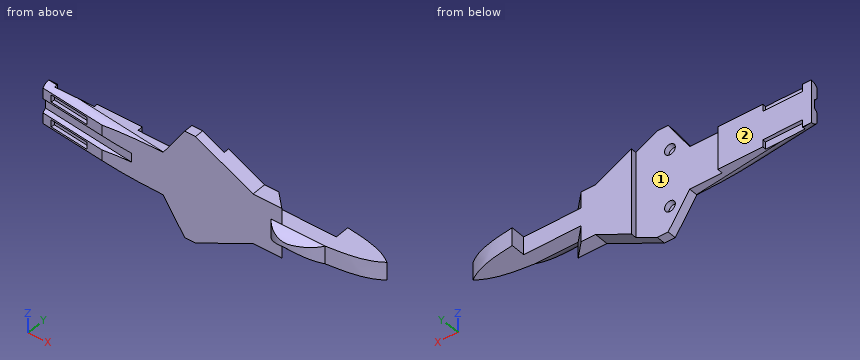
```python
from build123d import *

# Parameters (mm, degrees)
BOSS_EXTRUDE1_DEPTH     = 4
SKETCH2_R               = 1.5
BOSS_EXTRUDE2_DEPTH     = 3
CUT_EXTRUDE1_DEPTH      = 13
CUT_EXTRUDE2_DEPTH      = 49
CUT_EXTRUDE3_DEPTH      = 49
CUT_EXTRUDE3_DEPTH_BACK = 3
SKETCH5_R               = 1.5
CUT_EXTRUDE4_DEPTH      = 41
SKETCH7_W               = 11
SKETCH7_H               = 1
CUT_EXTRUDE5_DEPTH      = 2
CUT_EXTRUDE6_START      = -12
SKETCH7_2_W             = 11
SKETCH7_2_H             = 1
CUT_EXTRUDE6_DEPTH      = 2
SKETCH8_W               = 11
SKETCH8_H               = 2
CUT_EXTRUDE7_DEPTH      = 1
SKETCH9_W               = 14
SKETCH9_H               = 4
BOSS_EXTRUDE3_DEPTH     = 15
CUT_EXTRUDE8_DEPTH      = 15
SKETCH12_W              = 12
SKETCH12_H              = 4.5
CUT_EXTRUDE9_DEPTH      = 15
BOSS_EXTRUDE4_START     = -4.5
BOSS_EXTRUDE4_DEPTH     = 5
CUT_EXTRUDE10_DEPTH     = 4.5
CUT_EXTRUDE11_START     = -14
CUT_EXTRUDE11_DEPTH     = 4.5


with BuildPart() as part:
    # Sketch1 → Boss-Extrude1 (new body)
    with BuildSketch(Plane(origin=(0, 0, 0), x_dir=(1, 0, 0), z_dir=(0, 1, 0))):
        Polygon((-1, 15), (2, 15), (18, 7), (23, 7), (23, -7), (18, -7), (2, -15), (-1, -15), (-7, -6), (-42, -6), (-42, 6), (-7, 6), align=None)
    extrude(amount=BOSS_EXTRUDE1_DEPTH)

    # Sketch2 → Boss-Extrude2 (add)
    with BuildSketch(Plane(origin=(0, 4, 0), x_dir=(1, 0, 0), z_dir=(0, 1, 0))):
        with Locations(Location((-1.5, 8, 0), (0, 0, 270))):
            Circle(SKETCH2_R)
        with Locations(Location((-1.5, -8, 0), (0, 0, 90))):
            Circle(SKETCH2_R)
    extrude(amount=BOSS_EXTRUDE2_DEPTH)

    # Sketch3 → Cut-Extrude1 (cut)
    with BuildSketch(Plane.XY.offset(6)):
        Polygon((-24, 0), (-42, 2), (-42, 0), align=None)
    extrude(amount=-CUT_EXTRUDE1_DEPTH, mode=Mode.SUBTRACT)

    # Sketch4 → Cut-Extrude2 (cut, along a direction that is not the sketch's normal)
    with BuildSketch(Plane.ZY.offset(42)):
        with BuildLine():
            ThreePointArc((-5, 2), (-5.736067977, 2.881966011), (-6, 4))
            Line((-6, 4), (-6, 2))
            Line((-6, 2), (-5, 2))
        make_face()
        with BuildLine():
            Line((1.25, 2.910275264), (-1.25, 2.910275264))
            ThreePointArc((-1.25, 2.910275264), (-1.570550528, 2.410275264), (-2, 2))
            Line((-2, 2), (2, 2))
            ThreePointArc((2, 2), (1.570550528, 2.410275264), (1.25, 2.910275264))
        make_face()
        with BuildLine():
            Line((5, 2), (6, 2))
            Line((6, 2), (6, 4))
            ThreePointArc((6, 4), (5.736067977, 2.881966011), (5, 2))
        make_face()
    extrude(amount=-CUT_EXTRUDE2_DEPTH, dir=(-0.9938837346736189, 0.11043152607484653, 0), mode=Mode.SUBTRACT)

    # Sketch5 → Cut-Extrude3 (cut, two sides: drawn at the far end of the back side and taken through both)
    with BuildSketch(Plane(origin=(0, 4, 0), x_dir=(1, 0, 0), z_dir=(0, 1, 0)).offset(-CUT_EXTRUDE3_DEPTH_BACK)):
        with Locations(Location((-1.5, 8, 0), (0, 0, 270))):
            Circle(SKETCH5_R)
        with Locations(Location((-1.5, -8, 0), (0, 0, 270))):
            Circle(SKETCH5_R)
    extrude(amount=CUT_EXTRUDE3_DEPTH + CUT_EXTRUDE3_DEPTH_BACK, mode=Mode.SUBTRACT)

    # Sketch6 → Cut-Extrude4 (cut)
    with BuildSketch(Plane.XY.offset(15)):
        Polygon((-7, 4), (8, 4), (8, 2.5), (-7, 2.5), (-16, 2.5), (-16, 4), align=None)
    extrude(amount=-CUT_EXTRUDE4_DEPTH, mode=Mode.SUBTRACT)

    # Sketch7 → Cut-Extrude5 (cut)
    with BuildSketch(Plane.XY.offset(6)):
        with Locations((-34, 3.5)):
            Rectangle(SKETCH7_W, SKETCH7_H)
    extrude(amount=-CUT_EXTRUDE5_DEPTH, mode=Mode.SUBTRACT)

    # Sketch7<2> → Cut-Extrude6 (cut)
    with BuildSketch(Plane.XY.offset(6).offset(CUT_EXTRUDE6_START)):
        with Locations((-34, 3.5)):
            Rectangle(SKETCH7_2_W, SKETCH7_2_H)
    extrude(amount=CUT_EXTRUDE6_DEPTH, mode=Mode.SUBTRACT)

    # Sketch8 → Cut-Extrude7 (cut)
    with BuildSketch(Plane(origin=(-0.292682927, -2.634146341, 0), x_dir=(0.9938837346736189, -0.11043152607484653, 0), z_dir=(-0.11043152607484653, -0.9938837346736189, 0))):
        with Locations((-33.963979908, -3.5)):
            Rectangle(SKETCH8_W, SKETCH8_H)
        with Locations((-33.963979908, 3.5)):
            Rectangle(SKETCH8_W, SKETCH8_H)
    extrude(amount=-CUT_EXTRUDE7_DEPTH, mode=Mode.SUBTRACT)

    # Sketch9 → Boss-Extrude3 (add)
    with BuildSketch(Plane(origin=(23, 0, 0), x_dir=(0, 0, -1), z_dir=(1, 0, 0))):
        with Locations((0, 2)):
            Rectangle(SKETCH9_W, SKETCH9_H)
        with BuildLine():
            add(Edge.make_bspline(
                [(2.5, 0), (0.172282059, -6.003423798), (-2.5, 0)],
                knots=[0, 0, 0, 1, 1, 1], degree=2))
            Line((2.5, 0), (-2.5, 0))
        make_face()
    extrude(amount=BOSS_EXTRUDE3_DEPTH)

    # Sketch10 → Cut-Extrude8 (cut)
    with BuildSketch(Plane(origin=(0, 0, -7), x_dir=(-1, 0, 0), z_dir=(0, 0, -1))):
        with BuildLine():
            Line((-23, 0), (-23, -3.001711899))
            Line((-23, -3.001711899), (-38, -3.001711899))
            Line((-38, -3.001711899), (-38, 0))
            add(Edge.make_bspline(
                [(-23, 0), (-25.315557178, -3.079564153), (-31.097350972, -3.102014712), (-36.3128438, -1.382343261), (-38, 0)],
                knots=[0, 0, 0, 0, 0.604336881, 1, 1, 1, 1], degree=3))
        make_face()
    extrude(amount=-CUT_EXTRUDE8_DEPTH, mode=Mode.SUBTRACT)

    # Sketch12 → Cut-Extrude9 (cut)
    with BuildSketch(Plane.XZ):
        with Locations((32, -4.75)):
            Rectangle(SKETCH12_W, SKETCH12_H)
        with Locations((32, 4.75)):
            Rectangle(SKETCH12_W, SKETCH12_H)
    extrude(amount=-CUT_EXTRUDE9_DEPTH, mode=Mode.SUBTRACT)

    # Sketch10<4> → Boss-Extrude4 (add)
    with BuildSketch(Plane(origin=(0, 0, -7), x_dir=(-1, 0, 0), z_dir=(0, 0, -1)).offset(BOSS_EXTRUDE4_START)):
        with BuildLine():
            add(Edge.make_bspline(
                [(-38, 0), (-42.812604694, 0.581647057), (-48.098359819, 1.012932082), (-52.080952957, 4)],
                knots=[0, 0, 0, 0, 1, 1, 1, 1], degree=3))
            Line((-52.080952957, 4), (-38, 4))
            Line((-38, 4), (-38, 0))
        make_face()
        with BuildLine():
            Line((-52.080952957, 4), (-38, 4))
            Line((-38, 4), (-38, 8))
            add(Edge.make_bspline(
                [(-38, 8), (-42.812604694, 7.418352943), (-48.098359819, 6.987067918), (-52.080952957, 4)],
                knots=[0, 0, 0, 0, 1, 1, 1, 1], degree=3))
        make_face()
    extrude(amount=-BOSS_EXTRUDE4_DEPTH)

    # Sketch13 → Cut-Extrude10 (cut)
    with BuildSketch(Plane.XY.offset(7)):
        Polygon((22, 4), (26, 0), (26, 4), align=None)
    extrude(amount=-CUT_EXTRUDE10_DEPTH, mode=Mode.SUBTRACT)

    # Sketch13<2> → Cut-Extrude11 (cut)
    with BuildSketch(Plane.XY.offset(7).offset(CUT_EXTRUDE11_START)):
        Polygon((22, 4), (26, 0), (26, 4), align=None)
    extrude(amount=CUT_EXTRUDE11_DEPTH, mode=Mode.SUBTRACT)


solid = part.part
```
Geometry: final body of the model. Coordinates: model frame, mm. Face numbers are marked on the shaded views. Coordinates: 2 decimals unless noted, no trailing zeros. Order: outer loops, then holes, each group sorted by start corner. A loop starts at its lowest first (then second) coordinate and runs counter-clockwise, first axis right, second up. Notation, with made-up numbers: (11, 28.25) -> (31, 28.25) arc R19 ccw to (31, 37.25) -> close; hole circle Ø4 at (59.25, 33). An arc over 180 degrees is marked (long way). Write each question's results on one line, items separated by ' | '. Start each with the question number.
1) Cut plane A-A, the plane z = -8. Output: boundary loops of the cut face in (x, y), and give its area (3 significant figures).
2) Mould query, pull axis X, two halves, no side actions, for the marked faces 1 and 2. Classes: released by +X, released by -X, zero draft, split by the parting line, or undercut.
3) First-contact query: pin 1 (0.8 mm diameter, centred on x = -36, y = 3.5, fed in from -Z); pin 2 (0.8 mm diameter, centred on x = -31.5, y = 3.5, fed in from +Z); pin 3 (1.1 mm diameter, centred on y = 3.5, z = -5, fed in from +X). Flat tips, straight axial feed; report the tip coordinate or a pass-through.
4) Material intervals for line 1 along Z through (x, y) = (-1.5, 2.15); line 2 along Y through (x, z) = (9, 0); line 3 along Z through (x, y) = (27, 2.5), sorted ascending.
5) Cut plane C-C, the plane z = 13. Output: boundary loops of the cut face in (x, y), and give its area (3 significant figures).
6) Cut plane B-B, the plane x = 12. Output: boundary loops of the cut face in (y, z), and give its area (3 significant figures).
Checks:
1) outline: (-5.67, 0) -> (16, 0) -> (16, 4) -> (8, 4) -> (8, 2.5) -> (0, 2.5) -> (0, 1) -> (-3, 1) -> (-3, 2.5) -> (-5.67, 2.5) -> close | area: 61.7 mm^2
2) face 1: undercut | face 2: zero draft
3) pin 1: z = -4 | pin 2: z = 4 | pin 3: x = 23.05
4) line 1: -14.25 to -9.5, -6.5 to 6.5, 9.5 to 14.25 | line 2: 0 to 4 | line 3: -2.5 to 2.5
5) outline: (-2.33, 0) -> (6, 0) -> (6, 2.5) -> (-2.33, 2.5) -> close | area: 20.8 mm^2
6) outline: (0, -10) -> (4, -10) -> (4, 10) -> (0, 10) -> close | area: 80.0 mm^2
